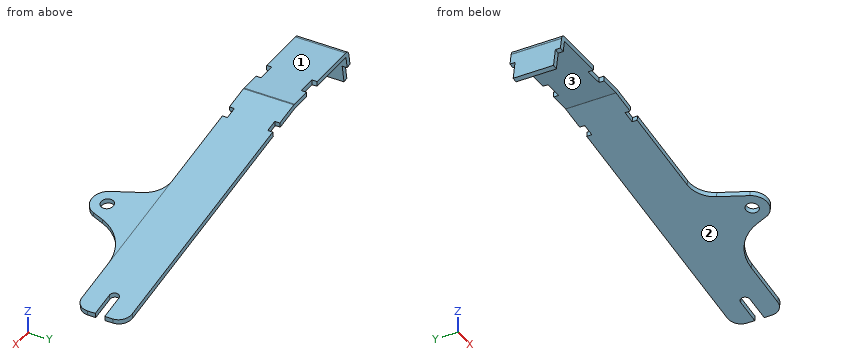
from build123d import *

# Parameters (mm, degrees)
SKETCH1_W               = 431.8
SKETCH1_H               = 50.8
BASE_FLANGE1_DEPTH      = 5.08
SKETCHED_START          = -25.4
SKETCHED_BEND1_DEPTH    = 50.8
SKETCHED_BEND1_2_DEPTH  = 50.8
SKETCHED_BEND2_DEPTH    = 50.8
SKETCHED_BEND2_2_DEPTH  = 50.8
SKETCH9_W               = 19.05
SKETCH9_H               = 5.08
CUT_EXTRUDE1_DEPTH      = 220.697648588
SKETCH10_W              = 19.05
SKETCH10_H              = 5.08
CUT_EXTRUDE2_DEPTH      = 398.423928706
SKETCH11_W              = 12.7
SKETCH11_H              = 5.08
CUT_EXTRUDE3_DEPTH      = 221.091320007
FILLET1_R               = 12.7
CUT_EXTRUDE4_DEPTH      = 221.036222152
CUT_EXTRUDE4_DEPTH_BACK = 221.036222152
SKETCH12_R              = 4.7625
SKETCH14_R              = 6.35
BOSS_EXTRUDE1_DEPTH     = 5.08
FILLET2_R               = 50.8
FILLET3_R               = 25.4


# Read off the part's stored shape, not the designer's step: Sketched Bend1, Sketched Bend2
# Sheet-metal steps are written as plain solids
with BuildPart() as part:
    # Sketch1 → Base-Flange1 (new body)
    with BuildSketch(Plane.XY):
        Rectangle(SKETCH1_W, SKETCH1_H)
    extrude(amount=-BASE_FLANGE1_DEPTH)

    # Sketched Bend1 outline → Sketched Bend1 (cut)
    with BuildSketch(Plane(origin=(0, 0, 0), x_dir=(1, 0, 0), z_dir=(0, 1, 0)).offset(SKETCHED_START)):
        with BuildLine():
            Line((-186.267525861, 4.80655801), (-186.315741061, 5.08))
            Line((-186.315741061, 5.08), (-215.9, 5.08))
            Line((-215.9, 5.08), (-215.9, 0))
            Line((-215.9, 0), (-180.539293085, 0))
            ThreePointArc((-180.539293085, 0), (-184.278131496, 1.360825892), (-186.267525861, 4.80655801))
        make_face()
    extrude(amount=SKETCHED_BEND1_DEPTH, mode=Mode.SUBTRACT)

    # Sketched Bend1 2 outline → Sketched Bend1 2 (add)
    with BuildSketch(Plane(origin=(0, 0, 0), x_dir=(1, 0, 0), z_dir=(0, 1, 0)).offset(SKETCHED_START)):
        with BuildLine():
            Line((-181.264702476, 5.688690752), (-186.61058496, 36.006696892))
            Line((-186.61058496, 36.006696892), (-191.613408345, 35.124564149))
            Line((-191.613408345, 35.124564149), (-186.315741061, 5.08))
            Line((-186.315741061, 5.08), (-180.539293085, 5.08))
            ThreePointArc((-180.539293085, 5.08), (-181.012770439, 5.252331663), (-181.264702476, 5.688690752))
        make_face()
    extrude(amount=SKETCHED_BEND1_2_DEPTH)

    # Sketched Bend2 outline → Sketched Bend2 (cut)
    with BuildSketch(Plane(origin=(0, 0, 0), x_dir=(1, 0, 0), z_dir=(0, 1, 0)).offset(SKETCHED_START)):
        with BuildLine():
            Line((215.9, 5.08), (-60.089888357, 5.08))
            Line((-60.089888357, 5.08), (-88.39884457, 0.088367224))
            ThreePointArc((-88.39884457, 0.088367224), (-88.901936467, 0.022133919), (-89.40888656, 0))
            Line((-89.40888656, 0), (215.9, 0))
            Line((215.9, 0), (215.9, 5.08))
        make_face()
    extrude(amount=SKETCHED_BEND2_DEPTH, mode=Mode.SUBTRACT)

    # Sketched Bend2 2 outline → Sketched Bend2 2 (add)
    with BuildSketch(Plane(origin=(0, 0, 0), x_dir=(1, 0, 0), z_dir=(0, 1, 0)).offset(SKETCHED_START)):
        with BuildLine():
            Line((210.826394713, 58.008217407), (-89.280977313, 5.091190609))
            ThreePointArc((-89.280977313, 5.091190609), (-89.34468764, 5.082802985), (-89.40888656, 5.08))
            Line((-89.40888656, 5.08), (-60.089888357, 5.08))
            Line((-60.089888357, 5.08), (211.708527455, 53.005394021))
            Line((211.708527455, 53.005394021), (210.826394713, 58.008217407))
        make_face()
    extrude(amount=SKETCHED_BEND2_2_DEPTH)

    # Sketch9 → Cut-Extrude1 (cut, through all)
    with BuildSketch(Plane(origin=(0, 0, -5.08), x_dir=(-1, 0, 0), z_dir=(0, 0, -1))):
        with Locations((120.214293085, 22.86)):
            Rectangle(SKETCH9_W, SKETCH9_H)
    cut_extrude1 = extrude(amount=-CUT_EXTRUDE1_DEPTH, mode=Mode.SUBTRACT)

    # Sketch10 → Cut-Extrude2 (cut, through all)
    with BuildSketch(Plane(origin=(-174.826079488, 0, 30.826554745), x_dir=(-0.17364817766692736, 0, -0.9848077530122086), z_dir=(0.9848077530122086, 0, -0.17364817766692736))):
        with Locations((58.339262271, 22.86)):
            Rectangle(SKETCH10_W, SKETCH10_H)
    cut_extrude2 = extrude(amount=-CUT_EXTRUDE2_DEPTH, mode=Mode.SUBTRACT)

    # Sketch11 → Cut-Extrude3 (cut, through all)
    with BuildSketch(Plane(origin=(-2.680663006, 0, -15.202795371), x_dir=(0.9848077530122081, 0, -0.17364817766693072), z_dir=(0.17364817766693072, 0, 0.9848077530122081))):
        with Locations((-55.290522683, 22.86)):
            Rectangle(SKETCH11_W, SKETCH11_H)
    cut_extrude3 = extrude(amount=-CUT_EXTRUDE3_DEPTH, mode=Mode.SUBTRACT)

    # Mirror1: Cut-Extrude1, Cut-Extrude2, Cut-Extrude3 across plane
    add(cut_extrude1.mirror(Plane.ZX), mode=Mode.SUBTRACT)
    add(cut_extrude2.mirror(Plane.ZX), mode=Mode.SUBTRACT)
    add(cut_extrude3.mirror(Plane.ZX), mode=Mode.SUBTRACT)

    # Fillet1
    fillet1_edges = [part.edges().sort_by_distance(p)[0] for p in [
        (211.267461084, 25.4, -55.506805714),
        (211.267461084, -25.4, -55.506805714),
    ]]
    fillet(fillet1_edges, radius=FILLET1_R)

    # Sketch12 → Cut-Extrude4 (cut, two sides: drawn at the far end of the back side and taken through both)
    with BuildSketch(Plane(origin=(-3.562795749, 0, -20.205618756), x_dir=(-0.9848077530122081, 0, 0.17364817766693072), z_dir=(-0.17364817766693072, 0, -0.9848077530122081)).offset(-CUT_EXTRUDE4_DEPTH_BACK)):
        with BuildLine():
            ThreePointArc((-192.296489295, -4.7625), (-197.058989295, 0), (-192.296489295, 4.7625))
            Line((-192.296489295, 4.7625), (-217.696489295, 4.7625))
            Line((-217.696489295, 4.7625), (-217.696489295, -4.7625))
            Line((-217.696489295, -4.7625), (-192.296489295, -4.7625))
        make_face()
        with Locations((-192.296489295, 0)):
            Circle(SKETCH12_R)
    extrude(amount=CUT_EXTRUDE4_DEPTH + CUT_EXTRUDE4_DEPTH_BACK, mode=Mode.SUBTRACT)

    # Sketch14 → Boss-Extrude1 (add)
    with BuildSketch(Plane(origin=(-3.562795749, 0, -20.205618756), x_dir=(-0.9848077530122081, 0, 0.17364817766693072), z_dir=(-0.17364817766693072, 0, -0.9848077530122081))):
        with BuildLine():
            Line((-75.889552591, -69.224530587), (-58.946489295, -25.4))
            Line((-58.946489295, -25.4), (-122.446489295, -25.4))
            Line((-122.446489295, -25.4), (-105.503425999, -69.224530587))
            ThreePointArc((-105.503425999, -69.224530587), (-90.696489295, -79.375), (-75.889552591, -69.224530587))
        make_face()
        with Locations((-90.696489295, -63.5)):
            Circle(SKETCH14_R, mode=Mode.SUBTRACT)
    extrude(amount=-BOSS_EXTRUDE1_DEPTH)

    # Fillet2
    fillet2_edges = [part.edges().sort_by_distance(p)[0] for p in [
        (117.46452261, -25.4, -38.966816791),
    ]]
    fillet(fillet2_edges, radius=FILLET2_R)

    # Fillet3
    # the kernel refuses this fillet: 25.4 mm, written as the material it adds along each edge
    with BuildSketch(Plane(origin=(54.488163922, -25.4, -30.441569202), x_dir=(0.35512202231381235, -0.9327204223089547, -0.06261759397767878), z_dir=(0.17364817766693072, 0, 0.9848077530122081))) as fillet3_piece_1:
        with BuildLine():
            CenterArc((FILLET3_R * 0.685521226707, -FILLET3_R), FILLET3_R, 90, 68.862929738)
            Line((-FILLET3_R * 0.247199195602, -FILLET3_R * 0.639399648076), (0, 0))
            Line((0, 0), (FILLET3_R * 0.685521226707, 0))
        make_face()
    extrude(amount=5.08)


solid = part.part
Verification items for the finished model (mm, model axes). Face numbers are marked on the shaded views. Give positions to 0.01 mm unless a question says otherwise; leave off trailing zeros. Write each loop counter-clockwise with the first axis right and the second up, starting at its lowest first coordinate (ties: lowest second). Pieces come first, ordered by that corner, then holes. Notation, with made-up numbers: M -15,-15 L 44,-15 A15 ccw 44,7 Z; hole C 54.25,81.5 d10. An arc over 180 degrees is marked long. Put each result on its own line as item: value. Start each with the question number.
1. Scan lines: line 1 along Y through (x, z) = (-94, -4); line 2 along Z through (x, y) = (175.5, -18.5); line 3 along Z through (x, y) = (15, 8.5). Record each from-to range of solid material in increasing order. Write a range as [from, to].
2. Section check A-A (x = -144.5). Record the cut outline in (y, z).
3. Section check B-B (y = -36.5). Record the cut outline in (x, z).
4. Draft check along X on the marked faces 1, 2 and 3. Enter one of: +X half, -X half, draft (parallel to the pull), parting line (faces both ways), or undercut.
5. Go/stop test with flat-tipped pins: pin 1 Ø6 at (x, z) = (-55, -7) entering from -Y; pin 2 Ø7.5 at (x, z) = (193, -52) entering from -Y; pin 3 Ø1.5 at (x, z) = (-119, -2.5) entering from +Y. Record where each tip stops, or that it passes through.
Answer list:
1. line 1: [-25.4, 25.4]
1. line 2: [-51.78, -46.62]
1. line 3: [-23.48, -18.32]
2. outline: M -25.4,-5.08 L 25.4,-5.08 L 25.4,0 L -25.4,0 Z
3. outline: M 58.01,-31.06 L 120.11,-42.01 L 120.99,-37.01 L 58.9,-26.06 Z
4. face 1: draft
4. face 2: undercut
4. face 3: undercut
5. pin 1: y = -20.32
5. pin 2: y = -25.4
5. pin 3: y = 20.32
